```python
from build123d import *

# Parameters (mm, degrees)
SKETCH1_R           = 3
BOSS_EXTRUDE1_DEPTH = 21


# Read off the part's stored shape, not the designer's step: M6x1.0 Machine Threads Stud1
with BuildPart() as part:
    # Sketch1 → Boss-Extrude1 (new, symmetric)
    with BuildSketch(Plane.XY):
        with Locations(Location((0, 0, 0), (0, 0, 180))):
            Circle(SKETCH1_R)
    extrude(amount=BOSS_EXTRUDE1_DEPTH, both=True)

    # M6x1.0 Machine Threads Stud1 outline → M6x1.0 Machine Threads Stud1 (revolve)
    with BuildSketch(Plane.XZ):
        Polygon((3, 21), (3, 30.4455), (2.4455, 31), (0, 31), (0, 21), align=None)
    m6x1_0_machine_threads_stud1 = revolve(axis=Axis((0, 0, 0), (0, 0, 1)))

    # Mirror1: M6x1.0 Machine Threads Stud1 across plane
    add(m6x1_0_machine_threads_stud1.mirror(Plane.XY))


solid = part.part
```
Here's how the part is built. I have some questions about the finished solid (model axes, mm). Round coordinates to 2 decimals unless told otherwise and drop trailing zeros. Order: outer loops, then holes, each group sorted by start corner. A loop starts at its lowest first (then second) coordinate and runs counter-clockwise, first axis right, second up. Notation, with made-up numbers: M -35,66 L -30,66 A27 ccw -30,89 Z; hole C 70.5,69 d5. An arc over 180 degrees is marked long. Use CSV: the item, a comma, the result in double quotes.
1) I want a section at A-A (z = 2.5). List the corners of the cut face in (x, y) for me.
Taken from the geometry:
outline,"C 0,0 d6"
2) I'm going to push flat-ended pins straight in: P1, Ø3, axis at y = 1.5, z = -12.5, coming from the +X side; P2, Ø1.5, axis at x = 1.5, z = -9, coming from the -Y side. Where does each tip first touch, or does it pass through?
Taken from the geometry:
P1,"x = 3"
P2,"y = -2.9"
3) I need wall thicknesses on line 1 along Y through (x, z) = (-0.1, -25); line 2 along X through (y, z) = (-2.2, -14.5); line 3 along Y through (x, z) = (0.75, -11.5). Which ranges of each line are inside material? Lowest first, please. Write a range as [from, to].
Taken from the geometry:
line 1,"[-3, 3]"
line 2,"[-2.04, 2.04]"
line 3,"[-2.9, 2.9]"
